Read the model definition and answer for the solid it produces. Units are mm, in the model's axes. A direction names the side the tool comes from. Coordinates: 2 decimals unless noted, no trailing zeros. Write each loop counter-clockwise with the first axis right and the second up, starting at its lowest first coordinate (ties: lowest second). Pieces come first, ordered by that corner, then holes. Notation, with made-up numbers: (65, 77) -> (119, 77) arc R33 ccw to (119, 110) -> close; hole circle Ø11 at (39, 49). An arc over 180 degrees is marked (long way). Answer as a JSON object with one key per item and string values. Group by question number.
(1) Find section B-B (z = 4.5). Give the vertices of the cut face in (x, y), then the cut area to 3 significant figures.
(2) Which of the six approach directions +Z, -Z, +X, -X, +Y, -Y give full straight-line access (tool end or side, diameter ignored) to faces 1 (the face through (0.2, 0.4, 7.5)), 2 (the face through (-1, 9, 0)), 3 (the face through (45, 2.7, 1.1)), 4 (the face through (45, 16, -6)), 5 (the face through (45, 16, 6))?
(3) Straight lines are drawn through the part: L1, parallel to X at y = 5, z = -1.5; L2, parallel to X at y = 3.5, z = -5.25; L3, parallel to Z at x = 40, y = 6.25. For each, find the intervals that lie inside material, in ascending order.
(4) Flat-ended cylindrical pins translate along their axes: P1, Ø2, axis at x = -6, y = 7.5, coming from the -Z side; P2, Ø0.8, axis at x = -44.5, z = 0, coming from the +Y side; P3, Ø1, axis at x = 43.5, z = -1.5, coming from the -Y side. Find the tip coordinate at first contact, or state that the pin passes through.
(5) For a pull along Y with two mould halves and no side action, classify faces 6 (the face through (55, 11, 0)), 7 (the face through (49.93, 17.82, 1.63)), 8 (the face through (1, 0.75, 0)) as +Y half, -Y half, draft (parallel to the pull), parting line (faces both ways), or undercut.
(6) Find section D-D (y = 16). Give the vertices of the cut face in (x, z).
(7) Find section A-A (x = -15). Give the vertices of the cut face in (y, z).
(8) Find section C-C (y = 6.5). Give the vertices of the cut face in (x, z), then the cut area to 3 significant figures.
Autodesk Inventor part; units mm, degrees
ref_plane "YZ Plane" through (0, 0, 0) normal (1, 0, 0) x (0, 1, 0)
ref_plane "XZ Plane" through (0, 0, 0) normal (0, 1, 0) x (-1, 0, 0)
ref_plane "XY Plane" through (0, 0, 0) normal (0, 0, 1) x (1, 0, 0)
sketch "Sketch1" plane through (0, 0, 0) normal (0, 1, 0) x (-1, 0, 0)
  line L0 (45, 7.5) -> (-45, 7.5)
  line L1 (-45, 7.5) -> (-45, -7.5)
  line L2 (-45, -7.5) -> (45, -7.5)
  line L3 (45, -7.5) -> (45, 7.5)
  line L4 (45, 7.5) -> (-45, -7.5) construction
  line L5 (-45, 7.5) -> (45, -7.5) construction
  point P0 (0, 0)
  dimension "d0" = 90
  dimension "d1" = 15
extrude "Plate1" add sketch "Sketch1" along normal blind 0.75
sketch "Sketch2" plane through (-44.25, 0, 7.5) normal (-1, 0, 0) x (0, -1, 0)
  line L0 (0, -15) -> (0, 0)
  line L1 (0, 0) -> (-14.5, 0)
  line L2 (-14.5, 0) -> (-14.5, -15)
  line L3 (-14.5, -15) -> (0, -15)
edge flange "Flange1" height 14.5 angle 90 thickness 0.75 bend radius 0.75 thickness toward (-1, 0, 0) relief tear relief width 0.75 relief depth 0.375 edges at (-45, 0.75, 0) wall of the first edge with corners at (-44.25, 0, -7.5) (-44.25, 0, 7.5) (-44.25, 14.5, 7.5) (-44.25, 14.5, -7.5)
bend "Bend1"
corner "Corner1"
sketch "Sketch3" plane through (44.25, 0, -7.5) normal (1, 0, 0) x (0, 1, 0)
  line L0 (0, 15) -> (0, 0)
  line L1 (0, 0) -> (18, 0)
  line L2 (18, 0) -> (18, 15)
  line L3 (18, 15) -> (0, 15)
edge flange "Flange2" height 18 angle 90 thickness 0.75 bend radius 0.75 thickness toward (1, 0, 0) relief tear relief width 0.75 relief depth 0.375 edges at (45, 0.75, 0) wall of the first edge with corners at (44.25, 0, 7.5) (44.25, 0, -7.5) (44.25, 18, -7.5) (44.25, 18, 7.5)
bend "Bend2"
corner "Corner2"
sketch "Sketch4" plane through (45, 18, 7.5) normal (1, 0, 0) x (0, 0, -1)
  circle A0 centre (7.5, -7.5) radius 7.5
  point P0 (7.5, -18)
  dimension "d23" = 10.5
  dimension "d24" = 15
extrude "Extrusion1" add sketch "Sketch4" along normal blind 10
sketch "Sketch5" plane through (-45, 14.5, -7.5) normal (-1, 0, 0) x (0, 0, 1)
  circle A0 centre (7.5, -4) radius 1.5
  circle A1 centre (12.5, -8) radius 1.5
  circle A2 centre (2.5, -8) radius 1.5
  point P0 (7.5, -14.5)
  dimension "d29" = 10.5
  dimension "d30" = 3
  dimension "d31" = 3
  dimension "d32" = 3
  dimension "d33" = 5
  dimension "d34" = 5
  dimension "d35" = 4
extrude "Extrusion2" add sketch "Sketch5" against normal up to surface (89.25 mm away)
equation "\"d34\" = d33"
equation "\"d2\" = Thickness"
equation "\"d3\" = BendReliefWidth"
equation "\"d4\" = BendReliefDepth"
equation "\"d5\" = MinimumRemnant"
equation "\"d6\" = TransitionRadius"
equation "\"d9\" = BendRadius"
equation "\"d10\" = CornerReliefSize"
equation "\"d11\" = GapSize"
equation "\"d12\" = JacobiRadiusSize"
equation "\"d13\" = BendReliefWidth"
equation "\"d14\" = BendReliefDepth"
equation "\"d15\" = MinimumRemnant"
equation "\"d16\" = TransitionRadius"
equation "\"d19\" = BendRadius"
equation "\"d20\" = CornerReliefSize"
equation "\"d21\" = GapSize"
equation "\"d22\" = JacobiRadiusSize"
equation "\"BendRadius\" = Thickness"
equation "\"BendReliefWidth\" = Thickness"
equation "\"BendReliefDepth\" = 0.5 * Thickness"
equation "\"CornerReliefSize\" = 4 * Thickness"
equation "\"MinimumRemnant\" = 2 * Thickness"
equation "\"TransitionRadius\" = BendRadius"
equation "\"JacobiRadiusSize\" = BendRadius"
equation "\"GapSize\" = Thickness"
properties part number "026" material "Stainless Steel, 440C"
Results below:
{
 "1": {"outline": "(-45, 1.5) arc R1.5 ccw to (-43.5, 0) -> (43.5, 0) arc R1.5 ccw to (45, 1.5) -> (45, 4.5) -> (55, 4.5) -> (55, 16.5) -> (45, 16.5) -> (45, 18) -> (44.25, 18) -> (44.25, 7.91) -> (-44.25, 7.91) -> (-44.25, 14.5) -> (-45, 14.5) -> close; hole (-44.25, 1.5) arc R0.75 ccw to (-43.5, 0.75) -> (43.5, 0.75) arc R0.75 ccw to (44.25, 1.5) -> (44.25, 5.09) -> (-44.25, 5.09) -> close", "area": "460 mm2"},
 "2": {"face 1": "+Z, +X, -X, +Y, -Y", "face 2": "none", "face 3": "+X, -Y", "face 4": "-Z, +X, +Y", "face 5": "+Z, +X, +Y"},
 "3": {"L1": "x = -45 to -44.25, 44.25 to 55", "L2": "x = -45 to -44.25, 44.25 to 45", "L3": "z = -6.48 to -3.52, 3.52 to 6.48"},
 "4": {"P1": "stops at z = -6.5", "P2": "stops at y = 14.5", "P3": "stops at y = 0"},
 "5": {"face 6": "draft", "face 7": "parting line", "face 8": "undercut"},
 "6": {"outline": "(44.25, -7.5) -> (45, -7.5) -> (45, -5.1) -> (55, -5.1) -> (55, 5.1) -> (45, 5.1) -> (45, 7.5) -> (44.25, 7.5) -> close"},
 "7": {"outline": "(0, -7.5) -> (0.75, -7.5) -> (0.75, 7.5) -> (0, 7.5) -> close; circle Ø3 at (6.5, -5); circle Ø3 at (6.5, 5); circle Ø3 at (10.5, 0)"},
 "8": {"outline": "(-45, -7.5) -> (-44.25, -7.5) -> (-44.25, -6.5) -> (44.25, -6.5) -> (44.25, -7.5) -> (45, -7.5) -> (45, -6.34) -> (55, -6.34) -> (55, 6.34) -> (45, 6.34) -> (45, 7.5) -> (44.25, 7.5) -> (44.25, 6.5) -> (-44.25, 6.5) -> (-44.25, 7.5) -> (-45, 7.5) -> close; hole (-44.25, -3.5) -> (44.25, -3.5) -> (44.25, 3.5) -> (-44.25, 3.5) -> close", "area": "680 mm2"}
}
